from build123d import *

# Parameters (mm, degrees)
BOSS_EXTRUDE1_DEPTH  = 70
SKETCH2_R            = 1.5
CUT_EXTRUDE1_DEPTH   = 6
LPATTERN1_COUNT      = 4
LPATTERN1_PITCH      = 14
LPATTERN1_COUNT_DIR2 = 2
LPATTERN1_PITCH_DIR2 = 55
CIRPATTERN2_COUNT    = 6
SKETCH10_R           = 6.5
CUT_EXTRUDE4_DEPTH   = 10
SKETCH11_R           = 20.2
SKETCH11_R_2         = 1.5
SKETCH11_R_3         = 6.5
BOSS_EXTRUDE6_DEPTH  = 9
SKETCH12_W           = 70
SKETCH12_H           = 13.5
SKETCH12_R           = 2.5
BOSS_EXTRUDE7_DEPTH  = 6


with BuildPart() as part:
    # Sketch1 → Boss-Extrude1 (new body)
    with BuildSketch(Plane.XY):
        Polygon((0, 26.7), (0, 0), (72.2, 0), (72.2, 71.7), (66.2, 71.7), (66.2, 26.7), (55, 26.7), (55, 13.5), (61, 13.5), (61, 18.7), (66.2, 18.7), (66.2, 6), (6, 6), (6, 18.7), (11.2, 18.7), (11.2, 13.5), (17.2, 13.5), (17.2, 26.7), align=None)
    extrude(amount=BOSS_EXTRUDE1_DEPTH)

    # Sketch2 → Cut-Extrude1 (cut)
    with BuildSketch(Plane.ZY.offset(-66.2)):
        with Locations(Location((50.75, 51.5, 0), (0, 0, 270))):
            Circle(SKETCH2_R)
    cut_extrude1 = extrude(amount=-CUT_EXTRUDE1_DEPTH, mode=Mode.SUBTRACT)

    # Sketch3 → Cut-Revolve1 (revolve, cut)
    with BuildSketch(Plane.XZ.offset(-18.7)):
        with BuildLine():
            Line((61.1, 56), (66.1, 56))
            ThreePointArc((66.1, 56), (63.6, 58.5), (61.1, 56))
        make_face()
    cut_revolve1 = revolve(axis=Axis((61.1, 18.7, 56), (1, 0, 0)), mode=Mode.SUBTRACT)

    # LPattern1: Cut-Revolve1 4 × 2
    with Locations(*[(-j * LPATTERN1_PITCH_DIR2, 0, -i * LPATTERN1_PITCH) for i in range(LPATTERN1_COUNT) for j in range(LPATTERN1_COUNT_DIR2) if (i, j) != (0, 0)]):
        add(cut_revolve1, mode=Mode.SUBTRACT)

    # CirPattern2: Cut-Extrude1 ×6 about axis
    cirpattern2_axis = Axis((0, 51.5, 35), (1, 0, 0))
    for i in range(1, CIRPATTERN2_COUNT):
        add(cut_extrude1.rotate(cirpattern2_axis, i * 360 / CIRPATTERN2_COUNT), mode=Mode.SUBTRACT)

    # Sketch10 → Cut-Extrude4 (cut)
    with BuildSketch(Plane.ZY.offset(-66.2)):
        with Locations((35, 44.5)):
            Circle(SKETCH10_R)
    extrude(amount=-CUT_EXTRUDE4_DEPTH, mode=Mode.SUBTRACT)

    # Sketch11 → Boss-Extrude6 (add)
    with BuildSketch(Plane(origin=(72.2, 0, 0), x_dir=(0, 0, -1), z_dir=(1, 0, 0))):
        with Locations(Location((-35, 51.5, 0), (0, 0, 90))):
            Circle(SKETCH11_R)
        with Locations(Location((-42.875, 65.13990011, 0), (0, 0, 210))):
            Circle(SKETCH11_R_2, mode=Mode.SUBTRACT)
        with Locations(Location((-27.125, 65.13990011, 0), (0, 0, 150))):
            Circle(SKETCH11_R_2, mode=Mode.SUBTRACT)
        with Locations(Location((-19.25, 51.5, 0), (0, 0, 90))):
            Circle(SKETCH11_R_2, mode=Mode.SUBTRACT)
        with Locations(Location((-27.125, 37.86009989, 0), (0, 0, 90))):
            Circle(SKETCH11_R_2, mode=Mode.SUBTRACT)
        with Locations(Location((-35, 44.5, 0), (0, 0, 180))):
            Circle(SKETCH11_R_3, mode=Mode.SUBTRACT)
        with Locations(Location((-42.875, 37.86009989, 0), (0, 0, 90))):
            Circle(SKETCH11_R_2, mode=Mode.SUBTRACT)
        with Locations(Location((-50.75, 51.5, 0), (0, 0, 270))):
            Circle(SKETCH11_R_2, mode=Mode.SUBTRACT)
    extrude(amount=BOSS_EXTRUDE6_DEPTH)

    # Sketch12 → Boss-Extrude7 (add)
    with BuildSketch(Plane(origin=(0, 0, 70), x_dir=(0, 0, -1), z_dir=(1, 0, 0))):
        with Locations((35, 33.45)):
            Rectangle(SKETCH12_W, SKETCH12_H)
        with Locations(Location((10, 33.45, 0), (0, 0, 270))):
            Circle(SKETCH12_R, mode=Mode.SUBTRACT)
        with Locations(Location((60, 33.45, 0), (0, 0, 270))):
            Circle(SKETCH12_R, mode=Mode.SUBTRACT)
    extrude(amount=BOSS_EXTRUDE7_DEPTH)


solid = part.part
Geometry check sheet. Reference: the model listing, model coordinates, mm. A direction names the side the tool comes from. Give positions to 0.01 mm unless a question says otherwise; leave off trailing zeros. Write each loop counter-clockwise with the first axis right and the second up, starting at its lowest first coordinate (ties: lowest second). Pieces come first, ordered by that corner, then holes. Notation, with made-up numbers: (-19.75, 58) - (-13.75, 58) arc R4 cw to (-13.75, 65) - close; hole circle Ø10 at (-30, -14). An arc over 180 degrees is marked (long way). Put each result on its own line as item: value.
1. Sectioned sample at A-A, the plane z = 10. Enter the section's corners in (x, y).
Ans:
outline: (0, 0) - (72.2, 0) - (72.2, 71.7) - (66.2, 71.7) - (66.2, 26.7) - (55, 26.7) - (55, 13.5) - (61, 13.5) - (61, 18.7) - (66.2, 18.7) - (66.2, 6) - (6, 6) - (6, 18.7) - (11.2, 18.7) - (11.2, 13.5) - (17.2, 13.5) - (17.2, 26.7) - (6, 26.7) - (6, 30.95) - (0, 30.95) - close; (0, 35.95) - (6, 35.95) - (6, 40.2) - (0, 40.2) - close
2. Sectioned sample at D-D, the plane x = 10. Enter the section's corners in (y, z).
Ans:
outline: (0, 0) - (6, 0) - (6, 70) - (0, 70) - close; (18.7, 0) - (26.7, 0) - (26.7, 70) - (18.7, 70) - (18.7, 58.07) arc R2.07 cw to (18.7, 53.93) - (18.7, 44.07) arc R2.07 cw to (18.7, 39.93) - (18.7, 30.07) arc R2.07 cw to (18.7, 25.93) - (18.7, 16.07) arc R2.07 cw to (18.7, 11.93) - close
3. Thickness scan on line 1 (X direction, y = 16, z = 18.5); line 2 (X direction, y = 30, z = 49); line 3 (Y direction, x = 1.35, z = 60). Record the ranges inside material, lowest first.
Ans:
line 1: x = 0 to 6, 11.2 to 17.2, 55 to 61, 66.2 to 72.2
line 2: x = 0 to 6, 66.2 to 72.2
line 3: y = 0 to 30.95, 35.95 to 40.2
4. Sectioned sample at C-C, the plane y = 44.5. Enter the section's corners in (x, z).
Ans:
outline: (66.2, 0) - (72.2, 0) - (72.2, 16.05) - (81.2, 16.05) - (81.2, 28.5) - (66.2, 28.5) - close; (66.2, 41.5) - (81.2, 41.5) - (81.2, 53.95) - (72.2, 53.95) - (72.2, 70) - (66.2, 70) - close
5. Go/stop test with flat-tipped pins: pin 1 (4 mm diameter, centred on y = 65.14, z = 27.12, fed in from -X); pin 2 (1.5 mm diameter, centred on x = 54.5, z = 57, fed in from +Y); pin 3 (8 mm diameter, centred on y = 33.45, z = 10, fed in from +X). Record where each tip stops, or that it passes through.
Ans:
pin 1: stops at x = 66.2
pin 2: stops at y = 26.7
pin 3: stops at x = 72.2
6. Sectioned sample at B-B, the plane y = 33.45. Enter the section's corners in (x, z), plus the area to 3 significant figures.
Ans:
outline: (0, 0) - (6, 0) - (6, 7.5) - (0, 7.5) - close; (0, 12.5) - (6, 12.5) - (6, 57.5) - (0, 57.5) - close; (0, 62.5) - (6, 62.5) - (6, 70) - (0, 70) - close; (66.2, 0) - (72.2, 0) - (72.2, 25.93) - (81.2, 25.93) - (81.2, 44.07) - (72.2, 44.07) - (72.2, 70) - (66.2, 70) - close
area: 943 mm²
7. Draft check along Z on faces 4 (the flat face through (57, 22, 0)), 5 (the flat face through (0, 20, 35)), 6 (the cylindrical face through (2.958, 31.065, 59.249)). Enter one of: +Z half, -Z half, draft (parallel to the pull), parting line (faces both ways), or undercut.
Ans:
face 4: -Z half
face 5: draft
face 6: undercut
8. Set-up check for faces 1 (the flat face through (58, 13.5, 35)), 2 (the flat face through (69, 71.7, 35)), 3 (the flat face through (6, 34, 35)): record each of +Z, -Z, +X, -X, +Y, -Y from which the full face is reachable in a straight line by a thin tool's end or side.
Ans:
face 1: +Z, -Z
face 2: +Z, -Z, +X, -X, +Y
face 3: +Z, -Z, +Y
